Could you check a few things on this model? Use its own coordinates, in mm. Face numbers are marked on the shaded views. A direction names the side the tool comes from. Coordinates: 2 decimals unless noted, no trailing zeros. Loops run counter-clockwise (first coordinate to the right, second up) from the corner with the lowest first, then second, coordinate; pieces in that order, holes last. Notation, with made-up numbers: (74.5, -21.5) -> (96.5, -21.5) arc R22 cw to (96.5, -1.5) -> close; hole circle Ø2 at (84.5, -10). An arc over 180 degrees is marked (long way). One line per question, with ' | ' between items. Start each with the question number.
(1) I'm going to push flat-ended pins straight in: pin 1 Ø6 at (x, y) = (12, -5) entering from -Z; pin 2 Ø5 at (x, z) = (-7, -6.5) entering from +Y; pin 3 Ø2.5 at (x, y) = (-15.5, -15.5) entering from -Z. Where does each tip first touch, or does it pass through?
(2) Suppose I cut it at C-C (z = 3). Please give me the cut outline in (x, y), plus the area to 3 significant figures.
(3) Suppose I cut it at D-D (y = 15.5). Please give me the cut outline in (x, z), plus the area to 3 significant figures.
(4) Which directions (+Z, -Z, +X, -X, +Y, -Y) give clear straight access to the entire face, cutting with the end or side of a thin tool? Please do the marked faces 5 and 6.
(5) If we mould it in two halves opening along X, with no side actions, what happens to the marked faces 1, 2, 3 and 4? For each: pulls with the +X half, pulls with the -X half, needs draft (parallel to the pull), parting line crosses it, or undercut.
(6) Suppose I cut it at A-A (x = 0). Please give me the cut outline in (y, z).
(7) Suppose I cut it at B-B (y = 0). Please give me the cut outline in (x, z).
(8) If I drill on line 1 along Y through (x, z) = (15.5, 4.25); line 2 along Z through (x, y) = (9, 14.5); line 3 along X through (y, z) = (7, 1.25), over which ranges is the centre line in solid material (lowest first)?
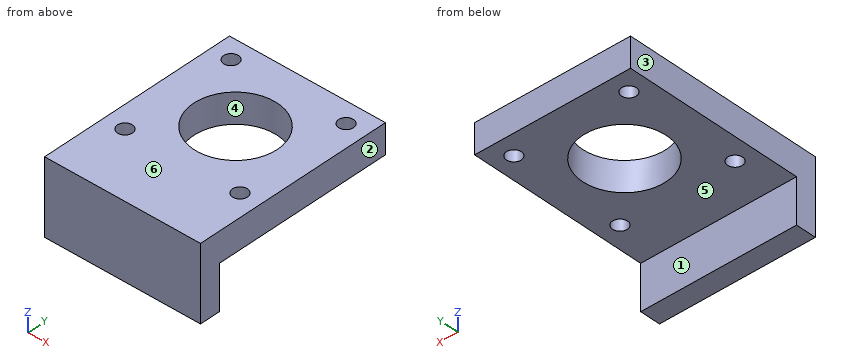
```python
from build123d import *

# Parameters (mm, degrees)
ESQUISSE1_W        = 42
ESQUISSE1_H        = 42
ESQUISSE1_R        = 2
ESQUISSE1_R_2      = 11.25
BOSS_EXTRU_1_DEPTH = 8
ESQUISSE2_W        = 42
ESQUISSE2_H        = 12
BOSS_EXTRU_2_DEPTH = 8
ESQUISSE3_W        = 42
ESQUISSE3_H        = 5.5
BOSS_EXTRU_3_DEPTH = 12


with BuildPart() as part:
    # Esquisse1 → Boss.-Extru.1 (new body)
    with BuildSketch(Plane.XY):
        Rectangle(ESQUISSE1_W, ESQUISSE1_H)
        with Locations((-15.5, 15.5)):
            Circle(ESQUISSE1_R, mode=Mode.SUBTRACT)
        with Locations((15.5, 15.5)):
            Circle(ESQUISSE1_R, mode=Mode.SUBTRACT)
        with Locations((15.5, -15.5)):
            Circle(ESQUISSE1_R, mode=Mode.SUBTRACT)
        with Locations((-15.5, -15.5)):
            Circle(ESQUISSE1_R, mode=Mode.SUBTRACT)
        Circle(ESQUISSE1_R_2, mode=Mode.SUBTRACT)
    extrude(amount=BOSS_EXTRU_1_DEPTH)

    # Esquisse2 → Boss.-Extru.2 (add)
    with BuildSketch(Plane.XY.offset(8)):
        with Locations((0, -27)):
            Rectangle(ESQUISSE2_W, ESQUISSE2_H)
    extrude(amount=-BOSS_EXTRU_2_DEPTH)

    # Esquisse3 → Boss.-Extru.3 (add)
    with BuildSketch(Plane(origin=(0, 0, 0), x_dir=(-1, 0, 0), z_dir=(0, 0, -1))):
        with Locations((0, -30.25)):
            Rectangle(ESQUISSE3_W, ESQUISSE3_H)
    extrude(amount=BOSS_EXTRU_3_DEPTH)


solid = part.part
```
Checks:
1) pin 1: stops at z = 0 | pin 2: stops at y = -27.5 | pin 3: passes through
2) outline: (-21, -33) -> (21, -33) -> (21, 21) -> (-21, 21) -> close; hole circle Ø4 at (-15.5, -15.5); hole circle Ø4 at (-15.5, 15.5); hole circle Ø22.5 at (0, 0); hole circle Ø4 at (15.5, -15.5); hole circle Ø4 at (15.5, 15.5) | area: 1,820 mm^2
3) outline: (-21, 0) -> (-17.5, 0) -> (-17.5, 8) -> (-21, 8) -> close; (-13.5, 0) -> (13.5, 0) -> (13.5, 8) -> (-13.5, 8) -> close; (17.5, 0) -> (21, 0) -> (21, 8) -> (17.5, 8) -> close | area: 272 mm^2
4) face 5: -Z, +X, -X, +Y | face 6: +Z, +X, -X, +Y, -Y
5) face 1: needs draft | face 2: pulls with the +X half | face 3: pulls with the -X half | face 4: undercut
6) outline: (-33, -12) -> (-27.5, -12) -> (-27.5, 0) -> (-11.25, 0) -> (-11.25, 8) -> (-33, 8) -> close; (11.25, 0) -> (21, 0) -> (21, 8) -> (11.25, 8) -> close
7) outline: (-21, 0) -> (-11.25, 0) -> (-11.25, 8) -> (-21, 8) -> close; (11.25, 0) -> (21, 0) -> (21, 8) -> (11.25, 8) -> close
8) line 1: y = -33 to -17.5, -13.5 to 13.5, 17.5 to 21 | line 2: z = 0 to 8 | line 3: x = -21 to -8.81, 8.81 to 21
